The listing builds one solid part. Answer for the finished solid, in the listing's coordinates (mm). Face numbers are marked on the shaded views. A direction names the side the tool comes from. Give positions to 0.01 mm unless a question says otherwise; leave off trailing zeros. Order: outer loops, then holes, each group sorted by start corner. A loop starts at its lowest first (then second) coordinate and runs counter-clockwise, first axis right, second up. Notation, with made-up numbers: (20.25, -15.5) - (56.25, -15.5) arc R12 cw to (56.25, -11.5) - close; hole circle Ø8 at (-16.75, -33). An arc over 180 degrees is marked (long way). Answer in a Markdown table with one row per item.
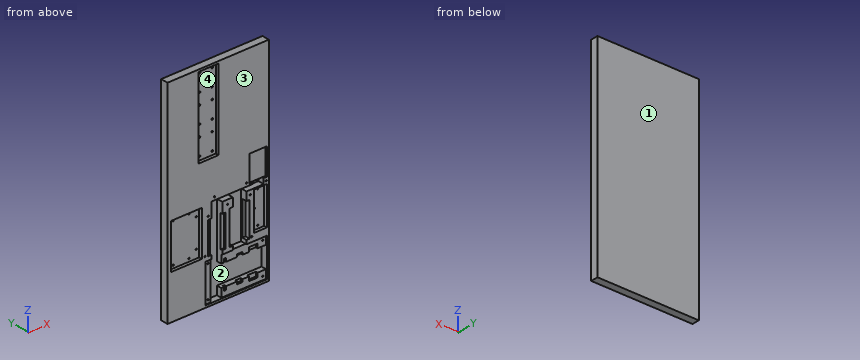
from build123d import *

# Parameters (mm, degrees)
SKETCH_1_W           = 23
SKETCH_1_H           = 80
EXTRUDE_1_DEPTH      = 7
SKETCH_1_5_W         = 19
SKETCH_1_5_H         = 76
CUT_EXTRUDE_2_DEPTH  = 3
SKETCH_2_R           = 0.75
CUT_EXTRUDE_3_DEPTH  = 2
SKETCH_4_W           = 96.2
SKETCH_4_H           = 80
EXTRUDE_2_DEPTH      = 7
SKETCH_5_W           = 29.4
SKETCH_5_H           = 42.4
SKETCH_5_W_2         = 12.4
SKETCH_5_H_2         = 36
CUT_EXTRUDE_4_DEPTH  = 3
SKETCH_6_R           = 0.65
CUT_EXTRUDE_5_DEPTH  = 2
SKETCH_8_W           = 96.2
SKETCH_8_H           = 7
EXTRUDE_3_DEPTH      = 40
SKETCH_15_W          = 27.5
SKETCH_15_H          = 80
SKETCH_15_W_2        = 45.7
EXTRUDE_4_DEPTH      = 7
SKETCH_9_W           = 58.2
SKETCH_9_H           = 36.2
CUT_EXTRUDE_6_DEPTH  = 1
SKETCH_10_W          = 1.7
SKETCH_10_H          = 26.6
SKETCH_10_W_2        = 5.2
SKETCH_10_H_2        = 25
SKETCH_10_W_3        = 8.1
SKETCH_10_H_3        = 28.2
SKETCH_10_W_4        = 3.1
SKETCH_10_H_4        = 20.2
CUT_EXTRUDE_7_DEPTH  = 2
SKETCH_11_R          = 0.65
CUT_EXTRUDE_8_DEPTH  = 2
SKETCH_12_W          = 16.4
SKETCH_12_H          = 30.2
CUT_EXTRUDE_9_DEPTH  = 1.7
SKETCH_13_W          = 19
SKETCH_13_H          = 32.2
CUT_EXTRUDE_10_DEPTH = 4.4
SKETCH_14_W          = 16.3
SKETCH_14_H          = 25.3
CUT_EXTRUDE_11_DEPTH = 1.7
SKETCH_16_W          = 10
SKETCH_16_H          = 4
SKETCH_16_W_2        = 6.1
SKETCH_16_W_3        = 13
SKETCH_16_H_2        = 32.2
SKETCH_16_W_4        = 10.4
SKETCH_16_H_3        = 30.2
SKETCH_16_H_4        = 3.6
SKETCH_16_W_5        = 42.4
SKETCH_16_H_5        = 20.2
CUT_EXTRUDE_12_DEPTH = 6
SKETCH_17_R          = 0.65
CUT_EXTRUDE_13_DEPTH = 3


with BuildPart() as part:
    # 草图1 → 凸台-拉伸1 (new body)
    with BuildSketch(Plane(origin=(0, 0, 0), x_dir=(1, 0, 0), z_dir=(0, 1, 0))):
        Rectangle(SKETCH_1_W, SKETCH_1_H)
    extrude(amount=EXTRUDE_1_DEPTH)

    # 草图1<5> → 切除-拉伸2 (cut)
    with BuildSketch(Plane(origin=(0, 0, 0), x_dir=(1, 0, 0), z_dir=(0, 1, 0))):
        Rectangle(SKETCH_1_5_W, SKETCH_1_5_H)
    extrude(amount=CUT_EXTRUDE_2_DEPTH, mode=Mode.SUBTRACT)

    # 草图2 → 切除-拉伸3 (cut)
    with BuildSketch(Plane.XZ.offset(-3)):
        with Locations(Location((-6, 34.580239709, 0), (0, 0, 270))):
            Circle(SKETCH_2_R)
        with Locations(Location((6, 34.580239709, 0), (0, 0, 270))):
            Circle(SKETCH_2_R)
        with Locations(Location((6, 18.580239709, 0), (0, 0, 270))):
            Circle(SKETCH_2_R)
        with Locations(Location((-6, 18.580239709, 0), (0, 0, 270))):
            Circle(SKETCH_2_R)
        with Locations(Location((-6, 8, 0), (0, 0, 270))):
            Circle(SKETCH_2_R)
        with Locations(Location((6, 8, 0), (0, 0, 270))):
            Circle(SKETCH_2_R)
        with Locations(Location((6, -8, 0), (0, 0, 270))):
            Circle(SKETCH_2_R)
        with Locations(Location((-6, -8, 0), (0, 0, 270))):
            Circle(SKETCH_2_R)
        with Locations(Location((-6, -18.580239709, 0), (0, 0, 270))):
            Circle(SKETCH_2_R)
        with Locations(Location((6, -18.580239709, 0), (0, 0, 270))):
            Circle(SKETCH_2_R)
        with Locations(Location((6, -34.580239709, 0), (0, 0, 270))):
            Circle(SKETCH_2_R)
        with Locations(Location((-6, -34.580239709, 0), (0, 0, 270))):
            Circle(SKETCH_2_R)
    extrude(amount=-CUT_EXTRUDE_3_DEPTH, mode=Mode.SUBTRACT)

    # 草图4 → 凸台-拉伸2 (add)
    with BuildSketch(Plane(origin=(0, 7, 0), x_dir=(1, 0, 0), z_dir=(0, 1, 0))):
        with Locations((9.1, 80)):
            Rectangle(SKETCH_4_W, SKETCH_4_H)
    extrude(amount=-EXTRUDE_2_DEPTH)

    # 草图5 → 切除-拉伸4 (cut)
    with BuildSketch(Plane.XZ):
        with Locations((-21.1, -97)):
            Rectangle(SKETCH_5_W, SKETCH_5_H)
        with Locations((49.2, -97)):
            Rectangle(SKETCH_5_W_2, SKETCH_5_H_2)
    extrude(amount=-CUT_EXTRUDE_4_DEPTH, mode=Mode.SUBTRACT)

    # 草图6 → 切除-拉伸5 (cut)
    with BuildSketch(Plane.XZ.offset(-3)):
        with Locations(Location((-31.1, -78.5, 0), (0, 0, 270))):
            Circle(SKETCH_6_R)
        with Locations(Location((-16.1, -78.5, 0), (0, 0, 270))):
            Circle(SKETCH_6_R)
        with Locations(Location((-31.1, -115.5, 0), (0, 0, 270))):
            Circle(SKETCH_6_R)
        with Locations(Location((-16.1, -115.5, 0), (0, 0, 270))):
            Circle(SKETCH_6_R)
        with Locations(Location((49.2, -112.273257218, 0), (0, 0, 270))):
            Circle(SKETCH_6_R)
        with Locations(Location((46.2, -97, 0), (0, 0, 270))):
            Circle(SKETCH_6_R)
        with Locations(Location((49.2, -81.726742782, 0), (0, 0, 270))):
            Circle(SKETCH_6_R)
        with Locations(Location((-9.1, -110.5, 0), (0, 0, 270))):
            Circle(SKETCH_6_R)
        with Locations(Location((-9.1, -83.5, 0), (0, 0, 270))):
            Circle(SKETCH_6_R)
    extrude(amount=-CUT_EXTRUDE_5_DEPTH, mode=Mode.SUBTRACT)

    # 草图8 → 凸台-拉伸3 (add)
    with BuildSketch(Plane(origin=(0, 0, -120), x_dir=(-1, 0, 0), z_dir=(0, 0, -1))):
        with Locations((-9.1, 3.5)):
            Rectangle(SKETCH_8_W, SKETCH_8_H)
    extrude(amount=EXTRUDE_3_DEPTH)

    # 草图15 → 凸台-拉伸4 (add, through all)
    with BuildSketch(Plane.XZ):
        with Locations((-25.25, 0)):
            Rectangle(SKETCH_15_W, SKETCH_15_H)
        with Locations((34.35, 0)):
            Rectangle(SKETCH_15_W_2, SKETCH_15_H)
    extrude(amount=-EXTRUDE_4_DEPTH)

    # 草图9 → 切除-拉伸6 (cut)
    with BuildSketch(Plane.XZ):
        with Locations((26.3, -139.9)):
            Rectangle(SKETCH_9_W, SKETCH_9_H)
    extrude(amount=-CUT_EXTRUDE_6_DEPTH, mode=Mode.SUBTRACT)

    # 草图10 → 切除-拉伸7 (cut)
    with BuildSketch(Plane.XZ.offset(-1)):
        with Locations((16.55, -139.9)):
            Rectangle(SKETCH_10_W, SKETCH_10_H)
        with Locations((30.6, -139.9)):
            Rectangle(SKETCH_10_W_2, SKETCH_10_H_2)
        with Locations((43.45, -139.9)):
            Rectangle(SKETCH_10_W_3, SKETCH_10_H_3)
        with Locations((53.85, -139.9)):
            Rectangle(SKETCH_10_W_4, SKETCH_10_H_4)
    extrude(amount=-CUT_EXTRUDE_7_DEPTH, mode=Mode.SUBTRACT)

    # 草图11 → 切除-拉伸8 (cut)
    with BuildSketch(Plane.XZ.offset(-1)):
        with Locations(Location((0.3, -124.9, 0), (0, 0, 270))):
            Circle(SKETCH_11_R)
        with Locations(Location((0.3, -154.9, 0), (0, 0, 270))):
            Circle(SKETCH_11_R)
        with Locations(Location((52.3, -154.9, 0), (0, 0, 270))):
            Circle(SKETCH_11_R)
        with Locations(Location((52.3, -124.9, 0), (0, 0, 270))):
            Circle(SKETCH_11_R)
    extrude(amount=-CUT_EXTRUDE_8_DEPTH, mode=Mode.SUBTRACT)

    # 草图12 → 切除-拉伸9 (cut)
    with BuildSketch(Plane.XZ):
        with Locations((7.8, -103.1)):
            Rectangle(SKETCH_12_W, SKETCH_12_H)
    extrude(amount=-CUT_EXTRUDE_9_DEPTH, mode=Mode.SUBTRACT)

    # 草图13 → 切除-拉伸10 (cut)
    with BuildSketch(Plane.XZ):
        with Locations((29.5, -102.1)):
            Rectangle(SKETCH_13_W, SKETCH_13_H)
    extrude(amount=-CUT_EXTRUDE_10_DEPTH, mode=Mode.SUBTRACT)

    # 草图14 → 切除-拉伸11 (cut)
    with BuildSketch(Plane.XZ):
        with Locations((47.25, -60.35)):
            Rectangle(SKETCH_14_W, SKETCH_14_H)
    extrude(amount=-CUT_EXTRUDE_11_DEPTH, mode=Mode.SUBTRACT)

    # 草图16 → 切除-拉伸12 (cut)
    with BuildSketch(Plane.XZ):
        Polygon((2.6, -74), (2.6, -88), (13, -88), (13, -78), (13, -74), align=None)
        with Locations((18, -76)):
            Rectangle(SKETCH_16_W, SKETCH_16_H)
        Polygon((23, -74), (23, -78), (23, -86), (36, -86), (36, -78), (36, -74), align=None)
        with Locations((39.05, -76)):
            Rectangle(SKETCH_16_W_2, SKETCH_16_H)
        Polygon((42.1, -73), (42.1, -74), (42.1, -78), (52.4, -78), (52.4, -73), align=None)
        with Locations((29.5, -102.1)):
            Rectangle(SKETCH_16_W_3, SKETCH_16_H_2)
        with Locations((7.8, -103.1)):
            Rectangle(SKETCH_16_W_4, SKETCH_16_H_3)
        with Locations((7.8, -120)):
            Rectangle(SKETCH_16_W_4, SKETCH_16_H_4)
        with Locations((29.5, -120)):
            Rectangle(SKETCH_16_W_3, SKETCH_16_H_4)
        Polygon((13, -121.8), (2.6, -121.8), (2.6, -158), (13, -158), (13, -150), (13, -129.8), align=None)
        with Locations((34.2, -139.9)):
            Rectangle(SKETCH_16_W_5, SKETCH_16_H_5)
    extrude(amount=-CUT_EXTRUDE_12_DEPTH, mode=Mode.SUBTRACT)

    # 草图17 → 切除-拉伸13 (cut)
    with BuildSketch(Plane.XZ):
        with Locations(Location((-3.4, -117.2, 0), (0, 0, 270))):
            Circle(SKETCH_17_R)
        with Locations(Location((41, -117.2, 0), (0, 0, 270))):
            Circle(SKETCH_17_R)
        with Locations(Location((-0.4, -85, 0), (0, 0, 270))):
            Circle(SKETCH_17_R)
        with Locations(Location((5.6, -71, 0), (0, 0, 270))):
            Circle(SKETCH_17_R)
        with Locations(Location((36.1, -71, 0), (0, 0, 270))):
            Circle(SKETCH_17_R)
        with Locations(Location((18, -82, 0), (0, 0, 270))):
            Circle(SKETCH_17_R)
        with Locations(Location((39.5, -82, 0), (0, 0, 270))):
            Circle(SKETCH_17_R)
        with Locations(Location((54.8, -76, 0), (0, 0, 270))):
            Circle(SKETCH_17_R)
    extrude(amount=-CUT_EXTRUDE_13_DEPTH, mode=Mode.SUBTRACT)


solid = part.part
Item 1: Find section B-B on x = 25. Write down the section's boundary in (y, z).
Answer block:
| item | result |
|---|---|
| outline | (0, -160) - (7, -160) - (7, 40) - (0, 40) - (0, -74) - (6, -74) - (6, -121.8) - (1, -121.8) - (1, -129.8) - (6, -129.8) - (6, -150) - (1, -150) - (1, -158) - (0, -158) - close |
Item 2: Find section A-A on z = -58. Write down the section's boundary in (x, y), then the cut area to 3 significant figures.
Answer block:
| item | result |
|---|---|
| outline | (-39, 0) - (39.1, 0) - (39.1, 1.7) - (55.4, 1.7) - (55.4, 0) - (57.2, 0) - (57.2, 7) - (-39, 7) - close |
| area | 646 mm² |
Item 3: Determine the mould class of the marked faces 1 and 2 for opening direction X: pulls with the +X half, pulls with the -X half, needs draft (parallel to the pull), parting line crosses it, or undercut.
Answer block:
| item | result |
|---|---|
| face 1 | needs draft |
| face 2 | undercut |
Item 4: Each of these flat-tipped pins is pushed along its axis until it touches: P1, Ø10, axis at x = 34, z = -26.5, coming from the -Y side; P2, Ø1, axis at x = 49, z = -81.5, coming from the -Y side; P3, Ø1.2, axis at x = 6, z = 18.5, coming from the -Y side. Where does it stop, or does it pass through?
Answer block:
| item | result |
|---|---|
| P1 | y = 0 |
| P2 | y = 3 |
| P3 | y = 5 |
Item 5: Which of the six approach directions +Z, -Z, +X, -X, +Y, -Y give full straight-line access (tool end or side, diameter ignored) to the marked faces 3 and 4?
Answer block:
| item | result |
|---|---|
| face 3 | +Z, -Z, +X, -X, -Y |
| face 4 | -Y |
Item 6: Consider line 1 (Z direction, x = 49.2, y = 3.5); line 2 (Z direction, x = 19, y = 2.25); line 3 (Z direction, x = 36.1, y = 1.6). Determine where each line is inside the solid, lowest interval first.
Answer block:
| item | result |
|---|---|
| line 1 | -160 to -150, -129.8 to -112.92, -111.62 to -82.38, -81.08 to -78, -73 to 40 |
| line 2 | -160 to -150, -129.8 to -78, -74 to 40 |
| line 3 | -160 to -150, -129.8 to -118.2, -86 to -78, -74 to -71.65, -70.35 to 40 |
